from build123d import *

# Parameters (mm, degrees)
F0_W     = 190.5
F0_H     = 21.746124
F1_DEPTH = 54.864
F3_W     = 190.5
F3_H     = 18.542
F4_DEPTH = 11.43
F6_W     = 190.5
F6_H     = 52.07
F7_DEPTH = 43.434
F8_W     = 190.5
F8_H     = 26.67
F9_DEPTH = 23.114


with BuildPart() as f1:
    # F0 (on Top) → F1 (new body)
    with BuildSketch(Plane.XY):
        Rectangle(F0_W, F0_H)
    extrude(amount=F1_DEPTH)

    # F3 (on face) → F4 (cut)
    with BuildSketch(Plane.XY.offset(54.864)):
        with Locations((0, -1.699938)):
            Rectangle(F3_W, F3_H)
    extrude(amount=-F4_DEPTH, mode=Mode.SUBTRACT)

    # F6 (on Top) → F7 (join)
    with BuildSketch(Plane.XY):
        with Locations((0, -15.161938)):
            Rectangle(F6_W, F6_H)
    extrude(amount=F7_DEPTH)

    # F8 (on face) → F9 (cut)
    with BuildSketch(Plane.XY.offset(54.864)):
        with Locations((0, -14.755538)):
            Rectangle(F8_W, F8_H)
    extrude(amount=-F9_DEPTH, mode=Mode.SUBTRACT)


solid = f1.part
Can you work these out from the model? Positions are in its coordinate system, mm. A direction names the side the tool comes from. Round coordinates to 2 decimals unless told otherwise and drop trailing zeros. Loops run counter-clockwise (first coordinate to the right, second up) from the corner with the lowest first, then second, coordinate; pieces in that order, holes last. Notation, with made-up numbers: (18.25, -13.5) - (28.25, -13.5) arc R8 cw to (28.25, 0.5) - close; hole circle Ø8 at (-29, 36.25). An arc over 180 degrees is marked (long way). Write item = value, one per line. Start each with the question number.
(1) If we mould it in two halves opening along Y, with no side actions, what happens to faces 1 (the face through (-1, -28.091, 38)), 2 (the face through (-1, -1.421, 38)), 3 (the face through (-1, 10.873, 27)), 4 (the face through (-1, -15, 0))? For each: released by +Y, released by -Y, zero draft, split by the parting line, or undercut.
(2) If we section it at A-A (z = 41): Please give me the cut outline in (x, y).
(3) For P1, Ø1, axis at x = -18.5, z = 49, coming from the -Y side; P2, Ø2.5, axis at x = -19.5, y = 4.5, coming from the +Z side; P3, Ø4, axis at x = 3, y = -9, coming from the +Z side, each with a flat end and sliding along its axis, tell me the tip position at first contact or that it passes through.
(4) For faces 5 (the face through (-95.25, -16, 21)), 6 (the face through (-1, -35, 43.434)), 7 (the face through (-1, -15, 31.75)), which set-ups out of +Z, -Z, +X, -X, +Y, -Y let a thin tool reach every point of the face, with its end or its side?
(5) If we section it at C-C (y = -36.5): Please give me the cut outline in (x, z).
(6) If we section it at D-D (z = 49.5): Please give me the cut outline in (x, y), and give its area (3 significant figures).
(7) If we section it at B-B (x = 25): Please give me the cut outline in (y, z).
(8) If I drill on probe 1 along Y at (x, z) = (-58.5, 36); probe 2 along Z at (x, y) = (-75, -28); probe 3 along Y at (x, z) = (32, 47), over which ranges is the centre line in solid material (lowest first)? Write a range as [from, to].
Ans:
q1.face_1 = undercut
q1.face_2 = undercut
q1.face_3 = released by +Y
q1.face_4 = zero draft
q2.outline = (-95.25, -41.2) - (95.25, -41.2) - (95.25, -28.09) - (-95.25, -28.09) - close; (-95.25, -1.42) - (95.25, -1.42) - (95.25, 10.87) - (-95.25, 10.87) - close
q3.P1 = 7.57
q3.P2 = 43.43
q3.P3 = 31.75
q4.face_5 = +Z, -Z, -X, +Y, -Y
q4.face_6 = +Z, +X, -X, -Y
q4.face_7 = +Z, +X, -X
q5.outline = (-95.25, 0) - (95.25, 0) - (95.25, 43.43) - (-95.25, 43.43) - close
q6.outline = (-95.25, 7.57) - (95.25, 7.57) - (95.25, 10.87) - (-95.25, 10.87) - close
q6.area = 629 mm²
q7.outline = (-41.2, 0) - (10.87, 0) - (10.87, 54.86) - (7.57, 54.86) - (7.57, 43.43) - (-1.42, 43.43) - (-1.42, 31.75) - (-28.09, 31.75) - (-28.09, 43.43) - (-41.2, 43.43) - close
q8.probe_1 = [-41.2, -28.09], [-1.42, 10.87]
q8.probe_2 = [0, 31.75]
q8.probe_3 = [7.57, 10.87]
